Autodesk Inventor part; units mm, degrees
ref_plane "YZ Plane" through (0, 0, 0) normal (1, 0, 0) x (0, 1, 0)
ref_plane "XZ Plane" through (0, 0, 0) normal (0, 1, 0) x (-1, 0, 0)
ref_plane "XY Plane" through (0, 0, 0) normal (0, 0, 1) x (1, 0, 0)
sketch "Sketch1" plane through (0, 0, 0) normal (0, 1, 0) x (-1, 0, 0)
  line L0 (5.8928, 5.8928) -> (-5.8928, 5.8928)
  line L1 (-5.8928, 5.8928) -> (-5.8928, -5.8928)
  line L2 (-5.8928, -5.8928) -> (5.8928, -5.8928)
  line L3 (5.8928, -5.8928) -> (5.8928, 5.8928)
  point P0 (0, 0)
  point P1 (5.8928, 0)
  point P2 (0, -5.8928)
  dimension "d0" = 11.7856
extrude "Extrusion1" add sketch "Sketch1" along normal blind 1.0668
sketch "Sketch2" plane through (0, 1.0668, 0) normal (0, 1, 0) x (1, 0, 0)
  line L0 (3.6703, -0.9779) -> (5.8928, -0.9779)
  line L1 (5.8928, -0.9779) -> (5.8928, 0.9779)
  line L2 (5.8928, 0.9779) -> (3.6703, 0.9779)
  line L3 (2.6924, 0) -> (2.6924, 0)
  line L4 (5.8928, -5.8928) -> (5.8928, 5.8928)
  arc A0 (3.6703, 0.9779) -> (2.6924, 0) centre (3.6703, 0) ccw
  arc A1 (2.6924, 0) -> (3.6703, -0.9779) centre (3.6703, 0) ccw
  line L5 (-0.9779, -5.8928) -> (0.9779, -5.8928)
  line L6 (0.9779, -5.8928) -> (0.9779, -3.6703)
  line L7 (0, -2.6924) -> (0, -2.6924)
  line L8 (-0.9779, -3.6703) -> (-0.9779, -5.8928)
  arc A2 (0.9779, -3.6703) -> (0, -2.6924) centre (0, -3.6703) ccw
  arc A3 (0, -2.6924) -> (-0.9779, -3.6703) centre (0, -3.6703) ccw
  line L9 (-5.8928, 5.8928) -> (-5.8928, -5.8928)
  line L10 (-5.8928, -0.9779) -> (-3.6703, -0.9779)
  line L11 (-2.6924, 0) -> (-2.6924, 0)
  line L12 (-3.6703, 0.9779) -> (-5.8928, 0.9779)
  line L13 (-5.8928, 0.9779) -> (-5.8928, -0.9779)
  arc A4 (-3.6703, -0.9779) -> (-2.6924, 0) centre (-3.6703, 0) ccw
  arc A5 (-2.6924, 0) -> (-3.6703, 0.9779) centre (-3.6703, 0) ccw
  line L14 (5.8928, 5.8928) -> (-5.8928, 5.8928)
  line L15 (-0.9779, 5.8928) -> (0.9779, 5.8928)
  line L16 (0.9779, 5.8928) -> (0.9779, 3.6703)
  line L17 (0, 2.6924) -> (0, 2.6924)
  line L18 (-0.9779, 3.6703) -> (-0.9779, 5.8928)
  arc A6 (-0.9779, 3.6703) -> (0, 2.6924) centre (0, 3.6703) ccw
  arc A7 (0, 2.6924) -> (0.9779, 3.6703) centre (0, 3.6703) ccw
  point P0 (0, 0)
  point P1 (2.6924, 0.9779)
  point P2 (2.6924, 0)
  point P3 (5.8928, 0)
  point P4 (5.8928, 0)
  point P5 (0.9779, -2.6924)
  point P6 (-0.9779, -2.6924)
  point P7 (0, -2.6924)
  point P8 (-2.6924, 0.9779)
  point P9 (-5.8928, 0)
  point P10 (-5.8928, 0)
  point P11 (0.9779, 2.6924)
  point P12 (0, 5.8928)
  point P13 (0, 5.8928)
  dimension "d3" = 3.2004
  dimension "d4" = 1.9558
  dimension "d5" = 0.9779
  dimension "d6" = 1.9558
  dimension "d7" = 3.2004
  dimension "d8" = 0.9779
  dimension "d9" = 3.2004
  dimension "d10" = 0.9779
  dimension "d11" = 3.2004
  dimension "d12" = 0.9779
extrude "Extrusion2" cut sketch "Sketch2" against normal blind 0.2794
fillet "Fillet1" radius 0.2794 12 edges at (-4.7816, 1.0668, 0.9779) (-4.7816, 1.0668, -0.9779) (-2.6924, 1.0668, 0) (0, 1.0668, -2.6924) (0.9779, 1.0668, -4.7816) (-0.9779, 1.0668, -4.7816) (2.6924, 1.0668, 0) (4.7816, 1.0668, 0.9779) (4.7816, 1.0668, -0.9779) (0, 1.0668, 2.6924) (-0.9779, 1.0668, 4.7816) (0.9779, 1.0668, 4.7816)
sketch "Sketch3" plane through (0, 0, 0) normal (0, -1, 0) x (1, 0, 0)
  point P0 (0, 0)
sketch "Sketch4" plane through (0, 1.0668, 0) normal (0, 1, 0) x (1, 0, 0)
  circle A0 centre (0, 0) radius 1.9685
  dimension "d16" = 3.937
extrude "Extrusion3" cut sketch "Sketch4" against normal through all
chamfer "Chamfer1" distance 0.0254 angle 45 16 edges at (5.8928, 1.0668, 3.5748) (5.8928, 0.9851, 1.0596) (3.5748, 1.0668, 5.8928) (1.0596, 0.9851, 5.8928) (5.8928, 1.0668, -3.5748) (5.8928, 0.9851, -1.0596) (3.5748, 1.0668, -5.8928) (1.0596, 0.9851, -5.8928) (-3.5748, 1.0668, -5.8928) (-1.0596, 0.9851, -5.8928) (-5.8928, 1.0668, -3.5748) (-5.8928, 0.9851, -1.0596) (-5.8928, 1.0668, 3.5748) (-5.8928, 0.9851, 1.0596) (-3.5748, 1.0668, 5.8928) (-1.0596, 0.9851, 5.8928)
chamfer "Chamfer2" distance 1.27 angle 45 4 edges at (5.8801, 1.0541, 5.8801) (5.8801, 1.0541, -5.8801) (-5.8801, 1.0541, -5.8801) (-5.8801, 1.0541, 5.8801)
fillet "Fillet2" radius 0.0254 4 edges at (-5.8928, 0.1318, 5.8928) (5.8928, 0.1318, 5.8928) (5.8928, 0.1318, -5.8928) (-5.8928, 0.1318, -5.8928)
properties part number "SSR-40 DA Big Plate" material "Nickel-Copper Alloy 400"
Source: CAD feature listing. Evaluate the final solid. Frame: model axes, mm. A direction names the side the tool comes from. Give positions to 0.01 mm unless a question says otherwise; leave off trailing zeros. Order: outer loops, then holes, each group sorted by start corner. A loop starts at its lowest first (then second) coordinate and runs counter-clockwise, first axis right, second up. Notation, with made-up numbers: (-19, 19) -> (3, 19) arc R5 ccw to (3, 23) -> close; hole circle Ø10 at (78.25, -14). An arc over 180 degrees is marked (long way). Use a Markdown table: item, result.
1) Contact query for flat-ended pins moving along their axis: P1, Ø2.5, axis at x = 0, z = 0, coming from the +Y side; P2, Ø1, axis at x = 4.5, z = 0, coming from the +Y side. Output: stop coordinate, or through.
Answer list:
| item | result |
|---|---|
| P1 | through |
| P2 | y = 0.79 |
2) Reachability of faces 4 (the flat face through (-4, 0.787, 0)), 5 (the flat face through (0, 0.787, -4)), 6 (the flat face through (0, 0.787, 4)) from +Z, -Z, +X, -X, +Y, -Y: full face, straight path, thin tool, end or side. Return the list, or none.
Answer list:
| item | result |
|---|---|
| face 4 | -X, +Y |
| face 5 | -Z, +Y |
| face 6 | +Z, +Y |
3) Ray query, line 1 along Z through (x, y) = (0, 0.3); line 2 along X through (y, z) = (0.9, 4.25); line 3 along Y through (x, z) = (-4.75, 0.5). Return the intervals inside material, ascending. Write a range as [from, to].
Answer list:
| item | result |
|---|---|
| line 1 | [-5.89, -1.97], [1.97, 5.89] |
| line 2 | [-5.89, -1], [1, 5.89] |
| line 3 | [0, 0.79] |
4) Section query C-C, the plane y = 0.5. Return the cut outline in (x, z), then the cut area to 3 significant figures.
Answer list:
| item | result |
|---|---|
| outline | (-5.89, -5.42) -> (-5.42, -5.89) -> (5.42, -5.89) -> (5.89, -5.42) -> (5.89, 5.42) -> (5.42, 5.89) -> (-5.42, 5.89) -> (-5.89, 5.42) -> close; hole circle Ø3.94 at (0, 0) |
| area | 126 mm² |
5) Mould query, pull axis Z, two halves, no side actions, for faces 1 (the flat face through (-5.39, 0.75, 5.42)), 2 (the flat face through (5.42, 0.75, -5.39)), 3 (the flat face through (4, 0.787, 0)). Classes: +Z half, -Z half, draft (parallel to the pull), parting line (faces both ways), or undercut.
Answer list:
| item | result |
|---|---|
| face 1 | +Z half |
| face 2 | -Z half |
| face 3 | undercut |
